Check sheet for the modelled part. Datum: model origin and axes. Units: mm. Face numbers are marked on the shaded views. A direction names the side the tool comes from. Round coordinates to 2 decimals unless told otherwise and drop trailing zeros. Write each loop counter-clockwise with the first axis right and the second up, starting at its lowest first coordinate (ties: lowest second). Pieces come first, ordered by that corner, then holes. Notation, with made-up numbers: (35.5, 87.25) -> (71.5, 87.25) arc R25 ccw to (71.5, 113.25) -> close; hole circle Ø11 at (26, 51.5). An arc over 180 degrees is marked (long way). Write item = value, one per line.
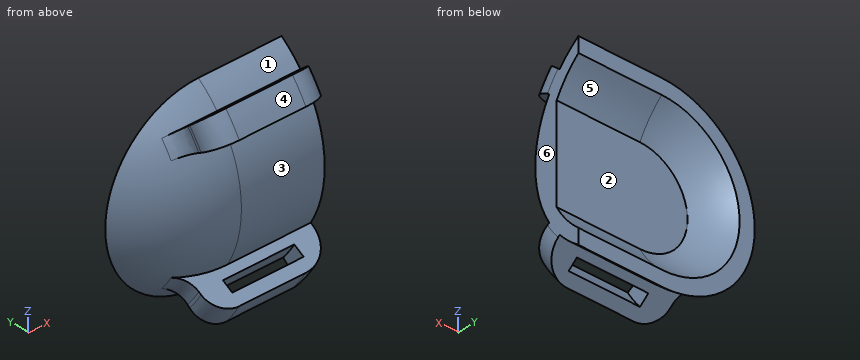
from build123d import *

# Parameters (mm, degrees)
SKETCH2_R                            = 12.2555
SKETCH2_R_2                          = 10.985499999999998
BOSS_EXTRUDE2_DEPTH                  = 15.239999999999998
CUT_EXTRUDE1_DEPTH                   = 24.079258231147723
CUT_EXTRUDE1_DEPTH_BACK              = 24.079258231147723
SKETCH6_W                            = 19.050000000000004
SKETCH6_H                            = 6.349999999999999
BOSS_EXTRUDE3_DEPTH                  = 11.43
BOSS_EXTRUDE3_DIRECTION_2_REACH      = 32.02
BOSS_EXTRUDE3_DIRECTION_2_END_RADIUS = 12.2555
SKETCH7_R                            = 1.4605000000000004
CUT_EXTRUDE3_DEPTH                   = 31.810720873585545
BOSS_EXTRUDE5_REACH                  = 32.02
LPATTERN1_COUNT                      = 3
LPATTERN1_PITCH                      = 5.334
CUT_EXTRUDE4_DEPTH                   = 35.034282139484006
FILLET5_R                            = 5.08
FILLET6_R                            = 2.54
BOSS_EXTRUDE6_REACH                  = 36.034
CUT_EXTRUDE5_DEPTH                   = 31.81072095045976
CUT_EXTRUDE5_DEPTH_BACK              = 31.81072095045976
CUT_EXTRUDE6_DEPTH                   = 31.81072095045976
CUT_EXTRUDE6_DEPTH_BACK              = 31.81072095045976
BOSS_EXTRUDE7_START                  = -12.7
BOSS_EXTRUDE7_DEPTH                  = 12.7
FILLET7_R                            = 2.286
FILLET8_R                            = 3.3019999999999996


with BuildPart() as part:
    # Sketch2 → Boss-Extrude2 (new body)
    with BuildSketch(Plane(origin=(0, 0, 0), x_dir=(0, 0, -1), z_dir=(1, 0, 0))):
        with Locations(Location((0, 0, 0), (0, 0, 180))):
            Circle(SKETCH2_R)
        with Locations(Location((0, 0, 0), (0, 0, 180))):
            Circle(SKETCH2_R_2, mode=Mode.SUBTRACT)
    extrude(amount=BOSS_EXTRUDE2_DEPTH)

    # Sketch3 → Revolve1 (revolve)
    with BuildSketch(Plane(origin=(0, 0, 0), x_dir=(1, 0, 0), z_dir=(0, 1, 0))):
        with BuildLine():
            Line((-12.2555, -1.5e-15), (-10.985499999999998, -1.35e-15))
            ThreePointArc((-10.985499999999998, 1.35e-15), (-7.767921544724782, 7.767921544724851), (9.58e-14, 10.985499999999998))
            Line((6.22e-15, 10.985499999999998), (6.94e-15, 12.2555))
            ThreePointArc((6.19e-15, 12.2555), (-8.665947156831733, 8.665947156831734), (-12.2555, 1.5e-15))
        make_face()
    revolve(axis=Axis((0, 0, 0), (-1, 0, 1.2e-16)))

    # Sketch4 → Cut-Extrude1 (cut, two sides: drawn at the far end of the back side and taken through both)
    with BuildSketch(Plane(origin=(0, 0, 0), x_dir=(1, 0, 0), z_dir=(0, 1, 0)).offset(-CUT_EXTRUDE1_DEPTH_BACK)):
        Polygon((15.239999999999998, 12.2555), (8.889999999999999, 12.255500000000001), (8.890000000000002, -12.255499999999998), (15.240000000000002, -12.2555), align=None)
    extrude(amount=CUT_EXTRUDE1_DEPTH + CUT_EXTRUDE1_DEPTH_BACK, mode=Mode.SUBTRACT)

    # Sketch6 → Boss-Extrude3 (add)
    with BuildSketch(Plane(origin=(0, 12.255499999999998, 0), x_dir=(1, 0, 0), z_dir=(0, 1, 0))):
        with Locations((-0.6349999999999953, 0)):
            Rectangle(SKETCH6_W, SKETCH6_H)
    extrude(amount=BOSS_EXTRUDE3_DEPTH)

    # Boss-Extrude3 direction 2: up to this cylinder (the profile starts outside it)
    boss_extrude3_direction_2_end = Plane(origin=(-0.6349999999999998, 0, 0), z_dir=(-1, 0, 0)) * Cylinder(BOSS_EXTRUDE3_DIRECTION_2_END_RADIUS, 89.551, mode=Mode.PRIVATE)
    # Sketch6 → Boss-Extrude3 direction 2 (add, up to the surface)
    with BuildSketch(Plane(origin=(0, 12.255499999999998, 0), x_dir=(1, 0, 0), z_dir=(0, 1, 0)), mode=Mode.PRIVATE) as boss_extrude3_direction_2_sk1:
        with Locations((-0.6349999999999953, 0)):
            Rectangle(SKETCH6_W, SKETCH6_H)
    boss_extrude3_direction_2_tool1 = extrude(boss_extrude3_direction_2_sk1.sketch, amount=-BOSS_EXTRUDE3_DIRECTION_2_REACH, mode=Mode.PRIVATE) - boss_extrude3_direction_2_end
    add(boss_extrude3_direction_2_tool1.solids().sort_by_distance((-0.635, 12.2555, 0))[0])
    add(boss_extrude3_direction_2_tool1.solids().sort_by_distance((-0.635, 12.2555, 0))[1])

    # Sketch7 → Cut-Extrude3 (cut, through all)
    with BuildSketch(Plane.XY.offset(3.175)):
        with Locations((4.889500000000005, 19.685)):
            Circle(SKETCH7_R)
    cut_extrude3 = extrude(amount=-CUT_EXTRUDE3_DEPTH, mode=Mode.SUBTRACT)

    # Sketch10 → Boss-Extrude5 (add, up to next)
    with BuildSketch(Plane(origin=(0, 12.255499999999998, 0), x_dir=(1, 0, 0), z_dir=(0, 1, 0)), mode=Mode.PRIVATE) as boss_extrude5_sk1:
        Polygon((8.83e-15, -3.175), (8.05e-15, 3.175), (-10.159999999999993, 3.175), (-10.159999999999997, -3.175), align=None)
    boss_extrude5_tool1 = extrude(boss_extrude5_sk1.sketch, amount=-BOSS_EXTRUDE5_REACH, mode=Mode.PRIVATE) - part.part
    add(boss_extrude5_tool1.solids().sort_by_distance((-5.08, 12.2555, 0))[0])

    # LPattern1: Cut-Extrude3 ×3
    with Locations(*[(-i * LPATTERN1_PITCH, 0, 0) for i in range(1, LPATTERN1_COUNT)]):
        add(cut_extrude3, mode=Mode.SUBTRACT)

    # Sketch8 → Cut-Extrude4 (cut, through all)
    with BuildSketch(Plane(origin=(8.89, 0, -1.26e-15), x_dir=(-1.1e-16, 0, -1), z_dir=(1, 0, -1.1e-16))):
        Polygon((-1.5875, 23.685499999999998), (1.5875, 23.685499999999998), (1.5874999999999988, 16.0655), (-1.5874999999999988, 16.0655), align=None)
    extrude(amount=-CUT_EXTRUDE4_DEPTH, mode=Mode.SUBTRACT)

    # Fillet5
    fillet5_edges = [part.edges().sort_by_distance(p)[0] for p in [
        (8.890000000000006, 23.685499999999998, 2.381249999999999),
        (-10.159999999999997, 23.685499999999998, -2.3812499999999996),
        (8.890000000000006, 23.685499999999998, -2.3812500000000005),
        (-10.159999999999997, 23.685499999999998, 2.3812500000000005),
    ]]
    fillet(fillet5_edges, radius=FILLET5_R)

    # Fillet6
    fillet6_edges = [part.edges().sort_by_distance(p)[0] for p in [
        (4.445000000000007, 11.83708812377436, -3.175),
        (4.445000000000007, 11.83708812377436, 3.175),
        (-5.840399850139422, 10.29594021158298, -3.175),
        (-5.840399850139422, 10.295940211582979, 3.175),
        (-10.159999999999995, 6.853588859130672, 4.2e-15),
    ]]
    fillet(fillet6_edges, radius=FILLET6_R)

    # Sketch11 → Boss-Extrude6 (add, up to next)
    with BuildSketch(Plane(origin=(8.89, 0, -1.26e-15), x_dir=(-1.5e-16, 0, -1), z_dir=(1, 0, -1.5e-16)), mode=Mode.PRIVATE) as boss_extrude6_sk1:
        with BuildLine():
            Line((5.08, -9.740370129004337), (-5.08, -9.740370129004337))
            ThreePointArc((-5.080000000000005, -9.740370129004335), (-3.31e-15, -10.985499999999998), (5.08, -9.740370129004337))
        make_face()
    boss_extrude6_tool1 = extrude(boss_extrude6_sk1.sketch, amount=-BOSS_EXTRUDE6_REACH, mode=Mode.PRIVATE) - part.part
    add(boss_extrude6_tool1.solids().sort_by_distance((8.89, -10.240924, 0))[0])

    # Sketch13 → Cut-Extrude5 (cut, two sides: drawn at the far end of the back side and taken through both)
    with BuildSketch(Plane.XY.offset(3.175).offset(-CUT_EXTRUDE5_DEPTH_BACK)):
        with BuildLine():
            Line((6.350000000000005, 14.795499999999999), (-1.2699999999999942, 14.7955))
            Line((-1.2699999999999942, 14.7955), (-1.2699999999999942, 13.587961408909038))
            ThreePointArc((-1.269999999999727, 13.587961408909017), (-0.6356900108532129, 13.632369326720188), (9.77e-15, 13.647182685448303))
            Line((1.089e-14, 13.647182685448303), (6.350000000000005, 13.647182685448303))
            Line((6.350000000000005, 13.647182685448303), (6.350000000000005, 14.795499999999999))
        make_face()
        with BuildLine():
            ThreePointArc((9.77e-15, 13.647182685448303), (-0.6356900108532129, 13.632369326720188), (-1.269999999999727, 13.587961408909017))
            Line((-1.2699999999999942, 13.587961408909038), (-1.269999999999994, 12.2555))
            Line((-1.269999999999994, 12.2555), (6.350000000000005, 12.2555))
            Line((6.350000000000005, 12.2555), (6.350000000000005, 13.647182685448303))
            Line((6.350000000000005, 13.647182685448303), (1.089e-14, 13.647182685448303))
        make_face()
    extrude(amount=CUT_EXTRUDE5_DEPTH + CUT_EXTRUDE5_DEPTH_BACK, mode=Mode.SUBTRACT)

    # Sketch14 → Cut-Extrude6 (cut, two sides: drawn at the far end of the back side and taken through both)
    with BuildSketch(Plane.XY.offset(3.175).offset(-CUT_EXTRUDE6_DEPTH_BACK)):
        Polygon((8.89, -7.175499999999997), (-12.255499999999998, -7.175499999999999), (-12.255500000000003, 23.685499999999998), (8.889999999999999, 23.685500000000005), align=None)
    extrude(amount=CUT_EXTRUDE6_DEPTH + CUT_EXTRUDE6_DEPTH_BACK, mode=Mode.SUBTRACT)

    # Sketch16 → Boss-Extrude7 (add)
    with BuildSketch(Plane(origin=(8.89, 0, -1.26e-15), x_dir=(-1.4e-16, 0, -1), z_dir=(1, 0, -1.4e-16)).offset(BOSS_EXTRUDE7_START)):
        with BuildLine():
            ThreePointArc((-7.397750000000142, -12.813278861692577), (-8.486350164031906, -12.119764071277773), (-9.510364079117075, -11.334010558166936))
            Line((-9.510364079117169, -11.334010558166854), (-10.153151688803709, -12.100055001285837))
            ThreePointArc((-10.153151688803714, -12.100055001285833), (-9.059926600382918, -12.93891611556679), (-7.89774999999997, -13.679304265477118))
            Line((-7.897749999999964, -13.679304265477123), (-7.397749999999962, -12.813278861692677))
        make_face()
        with BuildLine():
            ThreePointArc((-6.127749999999821, -10.61357433608029), (-7.029466015700107, -10.039117878783834), (-7.877683550513282, -9.38825767264472))
            Line((-7.877683550513363, -9.388257672644649), (-9.510364079117169, -11.334010558166854))
            ThreePointArc((-9.510364079117075, -11.334010558166936), (-8.486350164031906, -12.119764071277773), (-7.397750000000142, -12.813278861692577))
            Line((-7.397749999999962, -12.813278861692677), (-6.1277499999999705, -10.613574336080204))
        make_face()
        with BuildLine():
            ThreePointArc((-5.492750000000139, -9.513722073273868), (-6.301023941534394, -8.998794782536732), (-7.061343286211322, -8.415381229883662))
            Line((-7.06134328621146, -8.415381229883545), (-7.877683550513363, -9.388257672644649))
            ThreePointArc((-7.877683550513282, -9.38825767264472), (-7.029466015700107, -10.039117878783834), (-6.127749999999821, -10.61357433608029))
            Line((-6.1277499999999705, -10.613574336080204), (-5.492749999999971, -9.51372207327396))
        make_face()
        with BuildLine():
            ThreePointArc((7.061343286211319, -8.415381229883664), (6.3010239415344, -8.998794782536729), (5.492750000000143, -9.513722073273867))
            Line((5.492749999999974, -9.513722073273968), (6.127749999999969, -10.613574336080204))
            ThreePointArc((6.127749999999821, -10.613574336080289), (7.029466015700105, -10.039117878783832), (7.877683550513282, -9.388257672644716))
            Line((7.8776835505133604, -9.388257672644645), (7.061343286211458, -8.415381229883542))
        make_face()
        with BuildLine():
            ThreePointArc((7.877683550513282, -9.388257672644716), (7.029466015700105, -10.039117878783832), (6.127749999999821, -10.613574336080289))
            Line((6.127749999999969, -10.613574336080204), (7.397749999999963, -12.813278861692682))
            ThreePointArc((7.397750000000137, -12.81327886169258), (8.486350164031892, -12.119764071277785), (9.510364079117059, -11.33401055816695))
            Line((9.510364079117169, -11.334010558166854), (7.8776835505133604, -9.388257672644645))
        make_face()
        with BuildLine():
            ThreePointArc((9.510364079117059, -11.33401055816695), (8.486350164031892, -12.119764071277785), (7.397750000000137, -12.81327886169258))
            Line((7.397749999999963, -12.813278861692682), (7.897749999999962, -13.679304265477123))
            ThreePointArc((7.897749999999966, -13.679304265477121), (9.059926600382914, -12.938916115566794), (10.15315168880371, -12.100055001285837))
            Line((10.153151688803709, -12.100055001285837), (9.510364079117169, -11.334010558166854))
        make_face()
    extrude(amount=BOSS_EXTRUDE7_DEPTH)

    # Sketch17 → Cut-Revolve1 (revolve, cut)
    with BuildSketch(Plane(origin=(0, 0, 0), x_dir=(1, -7e-17, -8e-17), z_dir=(0, 0.6427876096865381, 0.7660444431189791))):
        Polygon((-1.269999999999997, -13.255499999999996), (6.350000000000001, -13.255499999999996), (6.350000000000001, -14.525499999999997), (-1.269999999999997, -14.525499999999996), align=None)
    revolve(axis=Axis((8.890000000000002, 0, 0), (-1, 0, 0)), mode=Mode.SUBTRACT)

    # Fillet7
    fillet7_edges = [part.edges().sort_by_distance(p)[0] for p in [
        (-3.809999999999998, -9.541668537674667, 6.681148237178193),
        (-3.8099999999999974, -12.938916115566784, 9.059926600382923),
        (-3.8099999999999996, -9.541668537674669, -6.681148237178193),
        (-3.81, -12.938916115566787, -9.059926600382923),
    ]]
    fillet(fillet7_edges, radius=FILLET7_R)

    # Fillet8
    fillet8_edges = [part.edges().sort_by_distance(p)[0] for p in [
        (8.890000000000002, -12.938916115566784, 9.059926600382921),
        (8.889999999999999, -12.938916115566787, -9.059926600382925),
    ]]
    fillet(fillet8_edges, radius=FILLET8_R)


solid = part.part
(1) Sectioned sample at C-C on x = 7.75. Enter the section's corners in (y, z), then the cut area to 3 significant figures.
Worked answers:
outline = (-12.98, -7.49) arc R14.99 ccw to (-11.48, -9.63) -> (-9.39, -7.88) arc R12.26 ccw to (-7.18, -9.94) -> (-7.18, -8.32) arc R10.99 cw to (-9.74, -5.08) -> (-9.74, 5.08) arc R10.99 cw to (-7.18, 8.32) -> (-7.18, 9.94) arc R12.26 ccw to (-9.39, 7.88) -> (-11.48, 9.63) arc R14.99 ccw to (-12.98, 7.49) -> (-10.61, 6.13) arc R12.26 ccw to (-10.61, -6.13) -> close
area = 48.2 mm²
(2) Release check for a two-part mould opening along Z. For the marked faces 4, 5 and 6 record: pulls with the +Z half, pulls with the -Z half, needs draft (parallel to the pull), parting line crosses it, or undercut.
Worked answers:
face_4 = pulls with the +Z half
face_5 = undercut
face_6 = needs draft
(3) Access from +Z, -Z, +X, -X, +Y, -Y to the whole of each face (thin tool, end or side, straight path). Record for the marked faces 1, 2 and 3.
Worked answers:
face_1 = +Z, +X, -X
face_2 = +X, +Y
face_3 = +X, -X, -Y
(4) Go/stop test with flat-tipped pins: P1, Ø0.7, axis at y = -11, z = -8, coming from the -X side; P2, Ø8, axis at x = -1.5, z = 0, coming from the +Y side; P3, Ø1, axis at x = 4, y = -12, coming from the -Z side; P4, Ø1.5, axis at x = 5, y = -10.5, coming from the -Z side. Record where each tip stops, or that it passes through.
Worked answers:
P1 = -3.81
P2 = -9.51
P3 = -10.15
P4 = -9.44
(5) Sectioned sample at D-D on z = 0.75. Enter the section's corners in (x, y), then the cut area to 3 significant figures.
Worked answers:
outline = (-9.91, -7.18) arc R12.23 ccw to (0, -12.23) -> (8.89, -12.23) -> (8.89, -9.74) -> (-5.02, -9.74) arc R10.96 cw to (-8.28, -7.18) -> close
area = 39.6 mm²
(6) Sectioned sample at A-A on x = 0.25. Enter the section's corners in (y, z), then the cut area to 3 significant figures.
Worked answers:
outline = (-13.68, -7.9) arc R15.8 ccw to (-12.1, -10.15) -> (-11.13, -9.34) arc R14.53 cw to (-12.58, -7.26) -> close; (-13.68, 7.9) -> (-12.58, 7.26) arc R14.53 cw to (-11.13, 9.34) -> (-12.1, 10.15) arc R15.8 ccw to start; (-11.48, -6.63) arc R13.26 ccw to (-10.15, -8.52) -> (-9.39, -7.88) arc R12.26 ccw to (-7.18, -9.94) -> (-7.18, -8.32) arc R10.99 cw to (-9.74, -5.08) -> (-9.74, 5.08) arc R10.99 cw to (-7.18, 8.32) -> (-7.18, 9.94) arc R12.26 ccw to (-9.39, 7.88) -> (-10.15, 8.52) arc R13.26 ccw to (-11.48, 6.63) -> (-10.61, 6.13) arc R12.26 ccw to (-10.61, -6.13) -> close
area = 46.4 mm²
(7) Sectioned sample at B-B on z = -3. Enter the section's corners in (x, y).
Worked answers:
outline = (-9.47, -7.18) arc R11.88 ccw to (0, -11.88) -> (8.89, -11.88) -> (8.89, -9.74) -> (-4.1, -9.74) arc R10.57 cw to (-7.76, -7.18) -> close
(8) Material ranges on L1, parallel to Z at x = -4.5, y = -8; L2, parallel to Z at x = -2.75, y = -10.75; L3, parallel to Z at x = -0.5, y = -12.5, recorded low to high. Write a range as [from, to].
Worked answers:
L1 = [-8.12, -6.04], [6.04, 8.12]
L2 = [-9.02, -6.21], [-5.2, 5.2], [6.21, 9.02]
L3 = [-9.66, -7.4], [7.4, 9.66]
